The listing builds one solid part. Answer for the finished solid, in the listing's coordinates (mm). Coordinates: 2 decimals unless noted, no trailing zeros. Order: outer loops, then holes, each group sorted by start corner. A loop starts at its lowest first (then second) coordinate and runs counter-clockwise, first axis right, second up.
```python
from build123d import *

# Parameters (mm, degrees)
ESQUISSE2_R = 1


with BuildPart() as part:
    # Balayage1: sweep along a path in Esquisse1
    with BuildLine(Plane.XY) as balayage1_path:
        Line((-4, 0), (-2, 0))
        ThreePointArc((-2, 0), (-0.585786438, -0.585786438), (0, -2))
        Line((0, -2), (0, -9))
        Line((0, -9), (-38.776114355, -292.440443433))
    # Esquisse2 → Balayage1 (sweep)
    with BuildSketch(Plane(origin=(-4, 0, 0), x_dir=(0, 0, -1), z_dir=(1, 0, 0))):
        Circle(ESQUISSE2_R)
    sweep(path=balayage1_path.line, transition=Transition.RIGHT)

    # Esquisse3 → Révolution1 (revolve)
    with BuildSketch(Plane.XY):
        Polygon((-4, 1), (-4, 2), (-3, 1), align=None)
    revolve(axis=Axis((0, 0, 0), (-1, 0, 0)))


solid = part.part
```
(1) Find section A-A (z = 0). Write down the section's boundary in (x, y), and give its area (3 significant figures).
(2) Consider line 1 (X direction, y = -124, z = 0.25); line 2 (X direction, y = -215.5, z = 0.4); line 3 (Z direction, x = -12.5, y = -96.5). Determine where each line is inside the solid, lowest interval first.
(3) Each of these flat-tipped pins is pushed along its axis until it touches: pin 1 Ø12 at (x, y) = (-18, -155.5) entering from +Z; pin 2 Ø2 at (y, z) = (-52.5, -1) entering from -X. Where does it stop, or does it pass through?
Findings below:
1. outline: (-39.77, -292.3) - (-37.79, -292.58) - (1, -9.07) - (1, -2) arc R3 ccw to (-2, 1) - (-3, 1) - (-4, 2) - (-4, -2) - (-3, -1) - (-2, -1) arc R1 cw to (-1, -2) - (-1, -8.93) - close
1. area: 597 mm2
2. line 1: x = -16.71 to -14.76
2. line 2: x = -29.18 to -27.33
2. line 3: z = -0.85 to 0.85
3. pin 1: stops at z = 1
3. pin 2: stops at x = -7.02
